Design review of the part built by this model. Coordinates are the model's own, in mm. Face numbers are marked on the shaded views. A direction names the side the tool comes from. Coordinates: 2 decimals unless noted, no trailing zeros. Write each loop counter-clockwise with the first axis right and the second up, starting at its lowest first coordinate (ties: lowest second). Pieces come first, ordered by that corner, then holes.
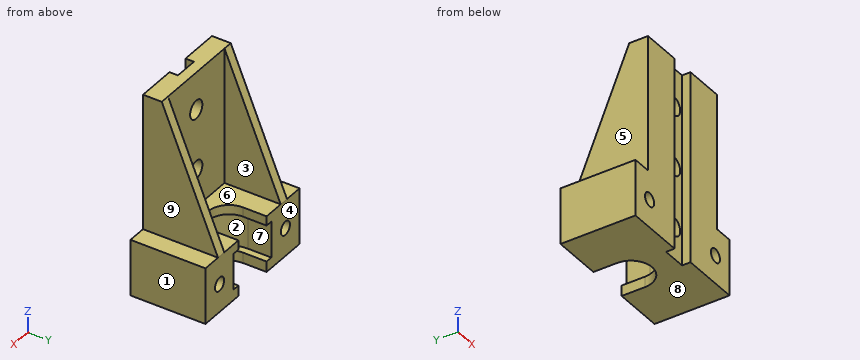
```python
from build123d import *

# Parameters (mm, degrees)
BOSS_EXTRUDE1_DEPTH = 12
CUT_EXTRUDE1_START  = -2
CUT_EXTRUDE1_DEPTH  = 7.75
SKETCH3_R           = 1.45
CUT_EXTRUDE2_DEPTH  = 18
BOSS_EXTRUDE2_DEPTH = 29
SKETCH5_R           = 1.95
CUT_EXTRUDE3_DEPTH  = 14.5
BOSS_EXTRUDE3_DEPTH = 2
BOSS_EXTRUDE4_START = -22
BOSS_EXTRUDE4_DEPTH = 2


with BuildPart() as part:
    # Sketch1 → Boss-Extrude1 (new body)
    with BuildSketch(Plane.XY):
        with BuildLine():
            Line((-5.280588843, 25), (-5.280588843, 41))
            Line((-5.280588843, 41), (5.219411157, 41))
            Line((5.219411157, 41), (5.219411157, 36))
            ThreePointArc((5.219411157, 36), (9.719411157, 31.5), (14.219411157, 36))
            Line((14.219411157, 36), (14.219411157, 41))
            Line((14.219411157, 41), (24.719411157, 41))
            Line((24.719411157, 41), (24.719411157, 25))
            Line((24.719411157, 25), (12.269411157, 25))
            Line((12.269411157, 25), (12.269411157, 26.8))
            Line((12.269411157, 26.8), (7.169411157, 26.8))
            Line((7.169411157, 26.8), (7.169411157, 25))
            Line((7.169411157, 25), (-5.280588843, 25))
        make_face()
    extrude(amount=-BOSS_EXTRUDE1_DEPTH)

    # Sketch2 → Cut-Extrude1 (cut)
    with BuildSketch(Plane.XY.offset(CUT_EXTRUDE1_START)):
        with BuildLine():
            Line((3.719411157, 36), (3.719411157, 41))
            Line((3.719411157, 41), (15.719411157, 41))
            Line((15.719411157, 41), (15.719411157, 36))
            ThreePointArc((15.719411157, 36), (9.719411157, 30), (3.719411157, 36))
        make_face()
    extrude(amount=-CUT_EXTRUDE1_DEPTH, mode=Mode.SUBTRACT)

    # Sketch3 → Cut-Extrude2 (cut)
    with BuildSketch(Plane(origin=(0, 41, 0), x_dir=(1, 0, 0), z_dir=(0, 1, 0))):
        with Locations((20.219411157, 6)):
            Circle(SKETCH3_R)
        with Locations((-0.780588843, 6)):
            Circle(SKETCH3_R)
    extrude(amount=-CUT_EXTRUDE2_DEPTH, mode=Mode.SUBTRACT)

    # Sketch4 → Boss-Extrude2 (add)
    with BuildSketch(Plane.XY):
        Polygon((-1.280588843, 25), (-1.280588843, 29), (20.719411157, 29), (20.719411157, 25), (12.269411157, 25), (12.269411157, 26.8), (7.169411157, 26.8), (7.169411157, 25), align=None)
    extrude(amount=BOSS_EXTRUDE2_DEPTH)

    # Sketch5 → Cut-Extrude3 (cut, symmetric)
    with BuildSketch(Plane(origin=(0, 29, 0), x_dir=(1, 0, 0), z_dir=(0, 1, 0))):
        with Locations((9.719411157, -21)):
            Circle(SKETCH5_R)
        with Locations((9.719411157, -8)):
            Circle(SKETCH5_R)
        with Locations((9.719411157, 5)):
            Circle(SKETCH5_R)
    extrude(amount=CUT_EXTRUDE3_DEPTH, both=True, mode=Mode.SUBTRACT)

    # Sketch6 → Boss-Extrude3 (add)
    with BuildSketch(Plane.ZY.offset(1.280588843)):
        Polygon((29, 29), (0, 41), (0, 29), align=None)
    extrude(amount=-BOSS_EXTRUDE3_DEPTH)

    # Sketch6<2> → Boss-Extrude4 (add)
    with BuildSketch(Plane.ZY.offset(1.280588843).offset(BOSS_EXTRUDE4_START)):
        Polygon((29, 29), (0, 41), (0, 29), align=None)
    extrude(amount=BOSS_EXTRUDE4_DEPTH)


solid = part.part
```
(1) Insertion check: pin 1 Ø6 at (x, z) = (9.72, -5) entering from -Y; pin 2 Ø8 at (y, z) = (31, 21) entering from +X; pin 3 Ø5 at (y, z) = (37, 14.5) entering from -X; pin 4 Ø2.5 at (x, z) = (-0.78, -6) entering from -Y. Each pin has a flat end and moves straight along its axis. Give the tip position at first contact, or say it passes through.
(2) For the marked faces 5, 6, 7, 8 and 9, list the 3-axis set-ups (+Z, -Z, +X, -X, +Y, -Y) from which the entire face can be reached by the end or side of a thin tool; tool diameter is ignored.
(3) Consider section A-A (y = 37). Give the boundary of the cut face in (x, z), plus the area to 3 significant figures.
(4) Consider section B-B (x = 9.5). Give the boundary of the cut face in (y, z).
(5) Consider section C-C (z = 8). Give the boundary of the cut face in (x, y).
(6) Mouldability with a two-part tool opening along X and no side actions: class the marked faces 1, 2, 3 and 4 as +X half, -X half, draft (parallel to the pull), parting line (faces both ways), or undercut.
(7) Consider section D-D (z = 0.5). Give the boundary of the cut face in (x, y), plus the area to 3 significant figures.
(8) Wall thickness on line 1 (X direction, y = 30, z = 23.5); line 2 (X direction, y = 28.55, z = 8); line 3 (X direction, y = 28.4, z = -5): over which ranges is each line inside the solid? List them lowest first.
Results:
1. pin 1: stops at y = 25
1. pin 2: stops at x = 20.72
1. pin 3: stops at x = -1.28
1. pin 4: passes through
2. face 5: +Z, -X, +Y, -Y
2. face 6: +Z, +Y
2. face 7: +Y
2. face 8: -Z, +X, -X, +Y, -Y
2. face 9: +Z, +X, +Y, -Y
3. outline: (-5.28, -12) - (5.22, -12) - (5.22, -9.75) - (3.72, -9.75) - (3.72, -2) - (5.22, -2) - (5.22, 0) - (0.72, 0) - (0.72, 9.67) - (-1.28, 9.67) - (-1.28, 0) - (-5.28, 0) - close; (14.22, -12) - (24.72, -12) - (24.72, 0) - (20.72, 0) - (20.72, 9.67) - (18.72, 9.67) - (18.72, 0) - (14.22, 0) - (14.22, -2) - (15.72, -2) - (15.72, -9.75) - (14.22, -9.75) - close; hole circle Ø2.9 at (-0.78, -6); hole circle Ø2.9 at (20.22, -6)
3. area: 254 mm2
4. outline: (26.8, -12) - (31.51, -12) - (31.51, -9.75) - (30, -9.75) - (30, -6.94) - (26.8, -6.94) - close; (26.8, -3.06) - (30, -3.06) - (30, -2) - (31.51, -2) - (31.51, 0) - (29, 0) - (29, 6.06) - (26.8, 6.06) - close; (26.8, 9.94) - (29, 9.94) - (29, 19.06) - (26.8, 19.06) - close; (26.8, 22.94) - (29, 22.94) - (29, 29) - (26.8, 29) - close
5. outline: (-1.28, 25) - (7.17, 25) - (7.17, 26.8) - (7.77, 26.8) - (7.77, 29) - (0.72, 29) - (0.72, 37.69) - (-1.28, 37.69) - close; (11.67, 26.8) - (12.27, 26.8) - (12.27, 25) - (20.72, 25) - (20.72, 37.69) - (18.72, 37.69) - (18.72, 29) - (11.67, 29) - close
6. face 1: +X half
6. face 2: undercut
6. face 3: undercut
6. face 4: draft
7. outline: (-1.28, 25) - (7.17, 25) - (7.17, 26.8) - (12.27, 26.8) - (12.27, 25) - (20.72, 25) - (20.72, 40.79) - (18.72, 40.79) - (18.72, 29) - (0.72, 29) - (0.72, 40.79) - (-1.28, 40.79) - close
7. area: 126 mm2
8. line 1: x = -1.28 to 0.72, 18.72 to 20.72
8. line 2: x = -1.28 to 7.77, 11.67 to 20.72
8. line 3: x = -5.28 to -1.83, 0.27 to 7.77, 11.67 to 19.17, 21.27 to 24.72
